Verification items for this drawing (mm, ordinates from the low corner). A direction names the side the tool comes from. Give positions to 0.01 mm unless a question says otherwise; leave off trailing zeros. Order: outer loops, then holes, each group sorted by start corner. A loop starts at its lowest first (then second) coordinate and runs counter-clockwise, first axis right, second up. Notation, with made-up numbers: (63.25, 9) -> (85.25, 9) arc R17 ccw to (85.25, 17) -> close; hole circle Ø9 at (38, 81). An arc over 180 degrees is marked (long way). One line per question, with ' | ' between items.
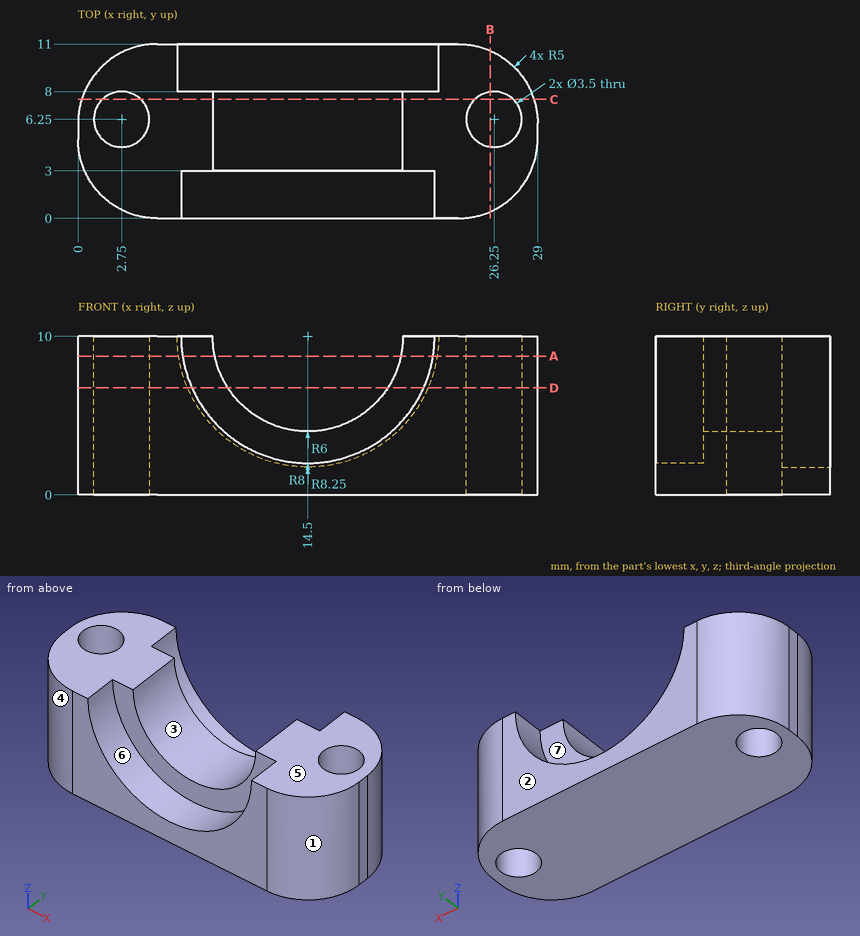
Q1. Section check A-A (z = 8.75). Enter the section's corners in (x, y), and give its area (3 significant figures).
Result sheet:
outline: (0, 5) arc R5 ccw to (5, 0) -> (6.6, 0) -> (6.6, 3) -> (8.63, 3) -> (8.63, 8) -> (6.35, 8) -> (6.35, 11) -> (5, 11) arc R5 ccw to (0, 6) -> close; (20.37, 3) -> (22.4, 3) -> (22.4, 0) -> (24, 0) arc R5 ccw to (29, 5) -> (29, 6) arc R5 ccw to (24, 11) -> (22.65, 11) -> (22.65, 8) -> (20.37, 8) -> close; hole circle Ø3.5 at (2.75, 6.25); hole circle Ø3.5 at (26.25, 6.25) | area: 123 mm2
Q2. Mould release check, pull along X, two halves, no side actions. Record for the marked faces 1, 2, 3 and 4: pulls with the +X half, pulls with the -X half, needs draft (parallel to the pull), parting line crosses it, or undercut.
Result sheet:
face 1: pulls with the +X half | face 2: needs draft | face 3: undercut | face 4: pulls with the -X half
Q3. Depth check by flat-ended pin: pin 1 Ø4 at (x, z) = (16, 5.5) entering from +Y; pin 2 Ø2 at (x, y) = (2.75, 6.25) entering from -Z; pin 3 Ø1 at (y, z) = (7.5, 2) entering from +X; pin 4 Ø4 at (x, z) = (26, 8.5) entering from -Y. Enter the tip coordinate at first touch or a pass-through.
Result sheet:
pin 1: stops at y = 8 | pin 2: passes through | pin 3: stops at x = 28.9 | pin 4: stops at y = 0
Q4. Section check B-B (x = 26). Enter the section's corners in (y, z).
Result sheet:
outline: (0.42, 0) -> (4.52, 0) -> (4.52, 10) -> (0.42, 10) -> close; (7.98, 0) -> (10.58, 0) -> (10.58, 10) -> (7.98, 10) -> close
Q5. Section check D-D (z = 6.75). Enter the section's corners in (x, y).
Result sheet:
outline: (0, 5) arc R5 ccw to (5, 0) -> (7.19, 0) -> (7.19, 3) -> (9.46, 3) -> (9.46, 8) -> (6.92, 8) -> (6.92, 11) -> (5, 11) arc R5 ccw to (0, 6) -> close; (19.54, 3) -> (21.81, 3) -> (21.81, 0) -> (24, 0) arc R5 ccw to (29, 5) -> (29, 6) arc R5 ccw to (24, 11) -> (22.08, 11) -> (22.08, 8) -> (19.54, 8) -> close; hole circle Ø3.5 at (2.75, 6.25); hole circle Ø3.5 at (26.25, 6.25)
Q6. Section check C-C (y = 7.5). Enter the section's corners in (x, z), and give its area (3 significant figures).
Result sheet:
outline: (0.23, 0) -> (1.53, 0) -> (1.53, 10) -> (0.23, 10) -> close; (3.97, 0) -> (25.03, 0) -> (25.03, 10) -> (20.5, 10) arc R6 cw to (8.5, 10) -> (3.97, 10) -> close; (27.47, 0) -> (28.77, 0) -> (28.77, 10) -> (27.47, 10) -> close | area: 180 mm2
Q7. Thickness scan on line 1 (X direction, y = 6.75, z = 6.5); line 2 (X direction, y = 5, z = 7.75); line 3 (Y direction, x = 20.75, z = 8.5). Record the ranges inside material, lowest first.
Result sheet:
line 1: x = 0.06 to 1.07, 4.43 to 9.63, 19.37 to 24.57, 27.93 to 28.94 | line 2: x = 0 to 1.53, 3.97 to 8.94, 20.06 to 25.03, 27.47 to 29 | line 3: y = 3 to 8
Q8. Access from +Z, -Z, +X, -X, +Y, -Y to the whole of each face (thin tool, end or side, straight path). Record for the marked faces 5, 6 and 7.
Result sheet:
face 5: +Z, +X, -X, +Y, -Y | face 6: +Z, -Y | face 7: +Z, +Y
